```python
from build123d import *

# Parameters (mm, degrees)
SKETCH1_R      = 3.3000188
SKETCH1_R_2    = 5.08
EXTRUDE1_DEPTH = 15.875
FILLET1_R      = 7.9375


with BuildPart() as part:
    # Sketch1 → Extrude1 (new body)
    with BuildSketch(Plane.XY):
        Polygon((174.8183702, 88.3592086), (131.1183814, 88.3896378), (131.1183814, 174.2591892), (174.8183702, 174.2591892), align=None)
        with Locations((166.9183606, 159.9092052)):
            Circle(SKETCH1_R, mode=Mode.SUBTRACT)
        with Locations((166.9183606, 102.7091926)):
            Circle(SKETCH1_R, mode=Mode.SUBTRACT)
        with Locations((142.2181814, 131.3091862)):
            Circle(SKETCH1_R_2, mode=Mode.SUBTRACT)
    extrude(amount=-EXTRUDE1_DEPTH)

    # Fillet1
    fillet1_edges = [part.edges().sort_by_distance(p)[0] for p in [
        (152.9683758, 88.3744232, -15.875),
        (152.9683758, 88.3744232, 0),
        (152.9683758, 174.2591892, -15.875),
        (152.9683758, 174.2591892, 0),
    ]]
    fillet(fillet1_edges, radius=FILLET1_R - 0.0001)  # a hair under: the kernel refuses the full size


solid = part.part
```
The model under review builds one solid part; all positions refer to its coordinate system, in mm. Give positions to 0.01 mm unless a question says otherwise; leave off trailing zeros. Write each loop counter-clockwise with the first axis right and the second up, starting at its lowest first coordinate (ties: lowest second). Pieces come first, ordered by that corner, then holes. Notation, with made-up numbers: (54.25, -30) -> (67.25, -30) arc R16 cw to (67.25, -23) -> close; hole circle Ø5 at (15, 59). An arc over 180 degrees is marked (long way). Put each result on its own line as item: value.
(1) We need section A-A, the plane z = -5.75. Give the boundary of the cut face in (x, y), and give its area (3 significant figures).
Results are:
outline: (131.12, 88.7) -> (174.82, 88.67) -> (174.82, 173.95) -> (131.12, 173.95) -> close; hole circle Ø10.16 at (142.22, 131.31); hole circle Ø6.6 at (166.92, 102.71); hole circle Ø6.6 at (166.92, 159.91)
area: 3,580 mm²
(2) The part is to be moulded in two halves that separate along Y. For faces 1 (the cylindrical face through (153.27, 172, -2.39)), 2 (the cylindrical face through (152.66, 90.64, -13.49)), 3 (the flat face through (131.118, 131, -8)), 4 (the cylindrical face through (138.2, 128.2, -7.8)), say which applies: pulls with the +Y half, pulls with the -Y half, needs draft (parallel to the pull), parting line crosses it, or undercut.
Results are:
face 1: pulls with the +Y half
face 2: pulls with the -Y half
face 3: needs draft
face 4: undercut
(3) To check wall thickness, follow probe 1 along Y at (x, z) = (168.5, -6.5); probe 2 along Y at (x, z) = (164, -6); probe 3 along X at (y, z) = (131.5, -13). State the ranges of each line that lie inside material, in increasing order. Write a range as from..to.
Results are:
probe 1: 88.49..99.81, 105.61..157.01, 162.81..174.13
probe 2: 88.61..101.17, 104.25..158.37, 161.45..174.02
probe 3: 131.12..137.14, 147.29..174.82
(4) We need section B-B, the plane y = 135. Give the boundary of the cut face in (x, z) (3 decimals).
Results are:
outline: (131.118, -15.875) -> (138.728, -15.875) -> (138.728, 0) -> (131.118, 0) -> close; (145.709, -15.875) -> (174.818, -15.875) -> (174.818, 0) -> (145.709, 0) -> close
(5) We need section C-C, the plane x = 168. State how many separate pieces and enclosed holes the cut face has, and give its area (3 significant figures).
Results are:
separate pieces: 3
enclosed holes: 0
area: 1,110 mm²
(6) We need section D-D, the plane z = -1. Give the boundary of the cut face in (x, y).
Results are:
outline: (131.12, 92.47) -> (174.82, 92.44) -> (174.82, 170.18) -> (131.12, 170.18) -> close; hole circle Ø10.16 at (142.22, 131.31); hole circle Ø6.6 at (166.92, 102.71); hole circle Ø6.6 at (166.92, 159.91)
(7) For pin 1 Ø5 at (x, z) = (149.5, -10.5) entering from -Y, flat-tipped, find the tip position at first contact; note if it passes through.
Results are:
pin 1: y = 88.38
